Design review of the part built by this model. Coordinates are the model's own, in mm. A direction names the side the tool comes from. Give positions to 0.01 mm unless a question says otherwise; leave off trailing zeros. Loops run counter-clockwise (first coordinate to the right, second up) from the corner with the lowest first, then second, coordinate; pieces in that order, holes last. Notation, with made-up numbers: M -38,57.25 L -3,57.25 A34 ccw -3,93.25 Z; hole C 27,3.25 d8. An arc over 180 degrees is marked long. Use one line per item in the form item = value. Start each with the question number.
Autodesk Inventor part; units mm, degrees
ref_plane "YZ Plane" through (0, 0, 0) normal (1, 0, 0) x (0, 1, 0)
ref_plane "XZ Plane" through (0, 0, 0) normal (0, 1, 0) x (-1, 0, 0)
ref_plane "XY Plane" through (0, 0, 0) normal (0, 0, 1) x (1, 0, 0)
sketch "Sketch1" plane through (0, 0, 0) normal (0, 0, 1) x (1, 0, 0)
  line L0 (-225, 200) -> (225, 200)
  line L1 (225, 200) -> (225, -200)
  line L2 (225, -200) -> (-225, -200)
  line L3 (-225, -200) -> (-225, 200)
  circle A0 centre (0, 0) radius 17.5
  point P0 (-225, 0)
  point P1 (0, 200)
  point P2 (-165, 104)
  dimension "d72" = 450
  dimension "d73" = 400
  dimension "d74" = 35
  dimension "d75" = 165
  dimension "d76" = 104
extrude "Extrusion1" add sketch "Sketch1" along normal blind 30 contours L0 L1 L2 L3 | A0
hole "Hole1" at (-165, 104, 0) direction (0, 0, 1) diameter 18 depth 30 counterbore diameter 26 counterbore depth 17.5
pattern_linear "Rectangular Pattern1" count 3 spacing 104 along (0, -1, 0) count 2 spacing 330 along (1, 0, 0) of "Hole1"
extrude "Extrusion2" [suppressed]
chamfer "Chamfer1" distance 0.5 angle 45 12 edges at (0, 200, 30) (-225, 0, 30) (-225, 200, 15) (-225, 0, 0) (0, 200, 0) (225, 200, 15) (225, 0, 30) (225, 0, 0) (225, -200, 15) (0, -200, 30) (0, -200, 0) (-225, -200, 15)
equation "\"d72\" = W_"
equation "\"d73\" = L"
equation "\"d74\" = dB"
equation "\"d77\" = H_"
equation "\"d79\" = S1_d1"
equation "\"d81\" = S1_d2"
equation "\"d82\" = S1_k"
equation "\"d84\" = H_"
equation "\"d92\" = H_"
equation "\"L\" = 400"
equation "\"W_\" = 450"
equation "\"H_\" = 30"
equation "\"S1_d1\" = 18"
equation "\"S1_d2\" = 26"
equation "\"S1_k\" = 17.5"
equation "\"S1_L\" = 208"
equation "\"dB\" = 35"
properties part number "SA-BCP-400x450x30x330" material "S 55 C"
Q1. For faces 5 (the cylindrical face through (-172.59, -99.16, 23.84)), 6 (the cylindrical face through (-152.31, 101.18, 8.87)), list the 3-axis set-ups (+Z, -Z, +X, -X, +Y, -Y) from which the entire face can be reached by the end or side of a thin tool; tool diameter is ignored.
Q2. Wall thickness on probe 1 along X at (y, z) = (0, 11.75); probe 2 along Y at (x, z) = (165, 27.25); probe 3 along Y at (x, z) = (-165, 6.25): over which ranges is each line inside the solid? List them lowest first.
Q3. Clearance check with flat-ended pins moving along their axes: pin 1 Ø21 at (x, y) = (161.5, -102) entering from -Z; pin 2 Ø23.5 at (x, y) = (165, 104) entering from -Z. State where each tip first meets the part, or that it passes through.
Q4. The part is to be moulded in two halves that separate along Y. For faces 1 (the flat face through (3, -200, 15)), 2 (the flat face through (-225, -3, 15)), 3 (the cylindrical face through (-152.31, -2.82, 8.87)), 4 (the flat face through (-174, 3, 17.5)), say which applies: pulls with the +Y half, pulls with the -Y half, needs draft (parallel to the pull), parting line crosses it, or undercut.
Q5. Take a section at A-A on y = -104. Give the boundary of the cut face in (x, z).
Response values:
q1.face_5 = +Z, -Z
q1.face_6 = -Z
q2.probe_1 = -225 to -178, -152 to 152, 178 to 225
q2.probe_2 = -200 to -113, -95 to -9, 9 to 95, 113 to 200
q2.probe_3 = -200 to -117, -91 to -13, 13 to 91, 117 to 200
q3.pin_1 = 0
q3.pin_2 = 17.5
q4.face_1 = pulls with the -Y half
q4.face_2 = needs draft
q4.face_3 = undercut
q4.face_4 = undercut
q5.outline = M -225,0.5 L -224.5,0 L -178,0 L -178,17.5 L -174,17.5 L -174,30 L -224.5,30 L -225,29.5 Z; M -156,17.5 L -152,17.5 L -152,0 L 152,0 L 152,17.5 L 156,17.5 L 156,30 L -156,30 Z; M 174,17.5 L 178,17.5 L 178,0 L 224.5,0 L 225,0.5 L 225,29.5 L 224.5,30 L 174,30 Z
